```python
from build123d import *

# Parameters (mm, degrees)
SKETCH_1_R           = 38
EXTRUDE_1_DEPTH      = 150
SKETCH_2_R           = 10
EXTRUDE_2_DEPTH      = 36
SKETCH_3_OUTSIDE_W   = 148.554
SKETCH_3_OUTSIDE_H   = 148.554
SKETCH_3_OUTSIDE_W_2 = 16
SKETCH_3_OUTSIDE_H_2 = 16
CUT_EXTRUDE_1_DEPTH  = 36


with BuildPart() as part:
    # 草图1 → 凸台-拉伸1 (new, symmetric)
    with BuildSketch(Plane.XY):
        Circle(SKETCH_1_R)
    extrude(amount=EXTRUDE_1_DEPTH, both=True)

    # 草图2 → 凸台-拉伸2 (add)
    with BuildSketch(Plane.XY.offset(150)):
        Circle(SKETCH_2_R)
    extrude_2 = extrude(amount=EXTRUDE_2_DEPTH)

    # 草图3 outside → 切除-拉伸1 (cut)
    with BuildSketch(Plane.XY.offset(186)):
        Rectangle(SKETCH_3_OUTSIDE_W, SKETCH_3_OUTSIDE_H)
        Rectangle(SKETCH_3_OUTSIDE_W_2, SKETCH_3_OUTSIDE_H_2, mode=Mode.SUBTRACT)
    cut_extrude_1 = extrude(amount=-CUT_EXTRUDE_1_DEPTH, mode=Mode.SUBTRACT)

    # 草图5 → M10 螺纹孔1 (revolve, cut)
    with BuildSketch(Plane(origin=(0, 8, 172), x_dir=(0, 0, 1), z_dir=(1, 0, 0))):
        Polygon((0, 0), (0, 27.053657631), (4.25, 24.5), (4.25, 1.275), (5.525, 0), align=None)
    hole_wizard_m10_1 = revolve(axis=Axis((0, 14.35, 172), (0, -1, 0)), mode=Mode.SUBTRACT)

    # 镜向1: 凸台-拉伸2, 切除-拉伸1, M10 螺纹孔1 across plane
    add(extrude_2.mirror(Plane.XY))
    add(cut_extrude_1.mirror(Plane.XY), mode=Mode.SUBTRACT)
    add(hole_wizard_m10_1.mirror(Plane.XY), mode=Mode.SUBTRACT)


solid = part.part
```
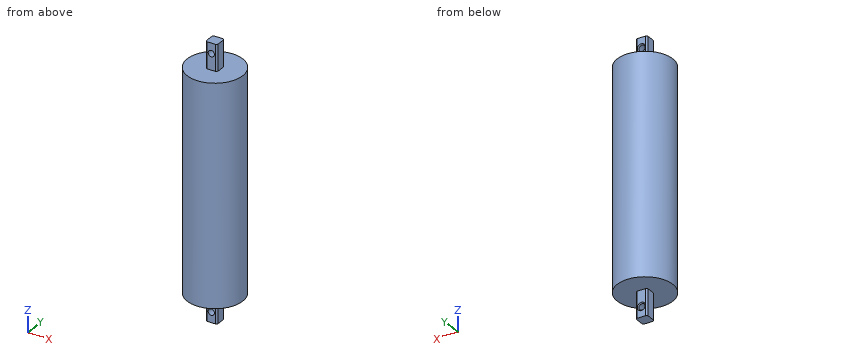
Can you work these out from the model? Positions are in its coordinate system, mm. Round coordinates to 2 decimals unless told otherwise and drop trailing zeros. Loops run counter-clockwise (first coordinate to the right, second up) from the corner with the lowest first, then second, coordinate; pieces in that order, holes last. Notation, with made-up numbers: M 48.25,24 L 75.25,24 A20 cw 75.25,59 Z; hole C 69,67 d2. An arc over 180 degrees is marked long. Answer as a JSON object with one key per item and string values. Group by question number.
Q1. Imagine slicing it at D-D, the plane z = 116.5. Please give me the cut outline in (x, y), then the cut area to 3 significant figures.
Q2. Imagine slicing it at C-C, the plane z = -172. Please give me the cut outline in (x, y) (3 decimals), then the cut area to 3 significant figures.
Q3. Imagine slicing it at B-B, the plane y = 0. Please give me the cut outline in (x, z), then the cut area to 3 significant figures.
Q4. Please list where these lines run through material, in increasing order: L1, parallel to Z at x = 0, y = 1; L2, parallel to X at y = 2.5, z = -172; L3, parallel to Z at x = -2.5, y = -3.
Q5. Imagine slicing it at A-A, the plane x = 0. Please give me the cut outline in (y, z) (3 decimals).
Q6. Will these pins go through, and if not, where does the flat tip stop? pin 1 (3.5 mm diameter, centred on x = -1, z = 160, fed in from -Y); pin 2 (3.5 mm diameter, centred on y = -2, z = 171.5, fed in from -X); pin 3 (4 mm diameter, centred on y = 6, z = -111.5, fed in from -X); pin 4 (5 mm diameter, centred on x = 0, z = 172, fed in from -Y).
Findings:
{
 "1": {"outline": "C 0,0 d76", "area": "4,540 mm2"},
 "2": {"outline": "M -8,-6 A10 ccw -6,-8 L -4.25,-8 L -4.25,6.725 L -5.525,8 L -6,8 A10 ccw -8,6 Z; M 4.25,-8 L 6,-8 A10 ccw 8,-6 L 8,6 A10 ccw 6,8 L 5.525,8 L 4.25,6.725 Z", "area": "111 mm2"},
 "3": {"outline": "M -38,-150 L -8,-150 L -8,-186 L 8,-186 L 8,-150 L 38,-150 L 38,150 L 8,150 L 8,186 L -8,186 L -8,150 L -38,150 Z; hole C 0,-172 d8.5; hole C 0,172 d8.5", "area": "23,800 mm2"},
 "4": {"L1": "z = -186 to -176.25, -167.75 to 167.75, 176.25 to 186", "L2": "x = -8 to -4.25, 4.25 to 8", "L3": "z = -186 to -175.44, -168.56 to 168.56, 175.44 to 186"},
 "5": {"outline": "M -38,-150 L -8,-150 L -8,-167.75 L 6.725,-167.75 L 8,-166.475 L 8,-150 L 38,-150 L 38,150 L 8,150 L 8,166.475 L 6.725,167.75 L -8,167.75 L -8,150 L -38,150 Z; M -8,-186 L 8,-186 L 8,-177.525 L 6.725,-176.25 L -8,-176.25 Z; M -8,176.25 L 6.725,176.25 L 8,177.525 L 8,186 L -8,186 Z"},
 "6": {"pin 1": "stops at y = -8", "pin 2": "stops at x = -8", "pin 3": "stops at x = -37.79", "pin 4": "passes through"}
}
